from build123d import *

# Parameters (mm, degrees)
F1_DEPTH = 25.4


with BuildPart() as f1:
    # F0 (on Top) → F1 (new body)
    with BuildSketch(Plane.XY):
        with BuildLine():
            ThreePointArc((-68.519122, 22.669713), (-95.134037, 0), (-68.519122, -22.669713))
            ThreePointArc((-68.519122, -22.669713), (-42.265052, -58.501721), (0, -72.171919))
            Line((0, -72.171919), (0, 72.171919))
            ThreePointArc((0, 72.171919), (-42.265052, 58.501721), (-68.519122, 22.669713))
        make_face()
    extrude(amount=F1_DEPTH)

    # F1_face (on face) → F2 (revolve)
    with BuildSketch(Plane(origin=(-35.565921, 0, 25.4), x_dir=(1, 0, 0), z_dir=(0, 0, 1))):
        with BuildLine():
            ThreePointArc((-32.953201, -22.669713), (-6.699131, -58.501721), (35.565921, -72.171919))
            Line((35.565921, -72.171919), (35.565921, 72.171919))
            ThreePointArc((35.565921, 72.171919), (-6.699131, 58.501721), (-32.953201, 22.669713))
            ThreePointArc((-32.953201, 22.669713), (-59.568116, 0), (-32.953201, -22.669713))
        make_face()
    revolve(axis=Axis((0, 0, 25.4), (0, 1, 0)))


solid = f1.part
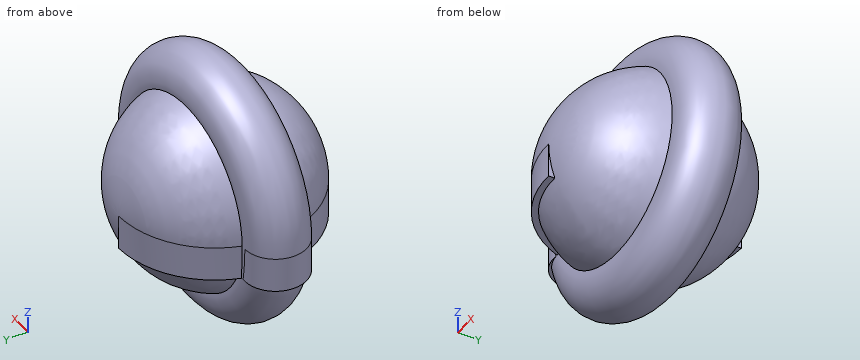
The listing builds one solid part. Answer for the finished solid, in the listing's coordinates (mm). Coordinates: 2 decimals unless noted, no trailing zeros. Write each loop counter-clockwise with the first axis right and the second up, starting at its lowest first coordinate (ties: lowest second). Pieces come first, ordered by that corner, then holes. Notation, with made-up numbers: M -32.75,28.5 L -7.75,28.5 A10 cw -7.75,32.5 Z; hole C 54,50.5 d9. An arc over 180 degrees is marked long. Write each question's results on one line, items separated by ' | '.
Item 1: Consider probe 1 along Y at (x, z) = (-58, 69); probe 2 along X at (y, z) = (-7, 24.5); probe 3 along Y at (x, z) = (-11, 5). Determine where each line is inside the solid, lowest interval first. Write a range as [from, to].
Answer below:
probe 1: [-22.96, 22.96] | probe 2: [-94.04, 94.04] | probe 3: [-71.33, 71.33]
Item 2: Given P1, Ø12, axis at x = -75.5, y = 10, coming from the +Z side; P2, Ø2, axis at y = -18, z = 56, coming from the -X side; P3, Ø1.5, axis at x = 51, z = 8, coming from the +Y side, each flat-ended and moving along its own axis, determine where each tip first touches the part or whether it passes through.
Answer below:
P1: z = 87.9 | P2: x = -82.15 | P3: y = 48.84
Item 3: The part is cut by section A-A on y = 7. Determine the outline of the cut face in (x, z).
Answer below:
outline: M -94.04,0 L -90.55,0 A94.04 ccw long -94.04,25.4 Z
